```python
from build123d import *

# Parameters (mm, degrees)
F1_W     = 123.9689588547
F1_H     = 36.4573895931
F1_W_2   = 0.162653625
F1_W_3   = 29.5906402171
F1_H_2   = 8.2422317937
F1_W_4   = 49.1941384971
F1_W_5   = 22.0608375967
F1_H_3   = 15.7345682383
F2_DEPTH = 38.1
F0_W     = 4.2057580379
F0_H     = 0.258524442
F0_H_2   = 4.8711853978
F0_W_2   = 4.3841055594
F0_H_3   = 57.6105192304
F3_DEPTH = 6.35


with BuildPart() as f2:
    # F1 (on Front) → F2 (new body)
    with BuildSketch(Plane.XZ):
        with Locations((29.8835039139, 199.447914958)):
            Rectangle(F1_W, F1_H)
        Polygon((-9.1060101986, 25.0596683472), (-9.1060101986, 20.0354661793), (2.2110529244, 20.0354661793), (2.2110529244, 76.3713121414), (-9.1060101986, 76.3713121414), align=None)
        Polygon((92.0306369662, 181.2192201614), (91.8679833412, 181.2192201614), (91.8679833412, 111.9364649057), (116.1640360951, 111.9364649057), (116.1640360951, 217.7610099316), (91.8679833412, 217.7610099316), (91.8679833412, 217.6766097546), (92.0306369662, 217.6766097546), align=None)
        with Locations((91.9493101537, 199.447914958)):
            Rectangle(F1_W_2, F1_H)
        Polygon((-87.8907889128, -68.0502578616), (-58.3001486957, -68.0502578616), (-58.3001486957, -42.4493700266), (-58.3001486957, 11.523572728), (-87.8907889128, 11.523572728), align=None)
        with Locations((-73.0954688042, 15.6446886249)):
            Rectangle(F1_W_3, F1_H_2)
        with BuildLine():
            Line((-9.1060101986, 19.7658045217), (-9.1060101986, 11.523572728))
            Line((-9.1060101986, 11.523572728), (0.2991169855, 11.523572728))
            ThreePointArc((0.2991169855, 11.523572728), (4.789245046, 13.3834446675), (6.6491169855, 17.873572728))
            Line((6.6491169855, 17.873572728), (6.6491169855, 20.0354661793))
            Line((6.6491169855, 20.0354661793), (2.2110529244, 20.0354661793))
            Line((2.2110529244, 20.0354661793), (-9.1060101986, 20.0354661793))
            Line((-9.1060101986, 20.0354661793), (-9.1060101986, 19.7658045217))
        make_face()
        with Locations((-33.7030794472, 15.6446886249)):
            Rectangle(F1_W_4, F1_H_2)
        with Locations((58.7894786149, 99.1525352001)):
            Rectangle(F1_W_5, F1_H_3)
        Polygon((69.8198974133, 91.285251081), (47.7590598166, 91.285251081), (47.7206557989, 91.285251081), (47.7206557989, 19.7658045217), (58.7702766061, 19.7658045217), (69.8198974133, 19.7658045217), align=None)
        Polygon((69.8198974133, -42.4493700266), (69.8198974133, 19.7658045217), (58.7702766061, 19.7658045217), (58.7702766061, 19.5491779596), (58.7702766061, -42.4493700266), align=None)
        Polygon((-58.3001486957, -68.0502578616), (69.8198974133, -68.0502578616), (69.8198974133, -42.4493700266), (58.7702766061, -42.4493700266), (-58.3001486957, -42.4493700266), align=None)
        Polygon((116.1640360951, 111.9364649057), (91.8679833412, 111.9364649057), (47.6743020117, 111.9364649057), (47.6743020117, 107.0198193192), (47.7590598166, 107.0198193192), (69.8198974133, 107.0198193192), (116.1640360951, 107.0198193192), align=None)
        Polygon((116.1640360951, -68.0502578616), (116.1640360951, 107.0198193192), (69.8198974133, 107.0198193192), (69.8198974133, 91.285251081), (69.8198974133, 19.7658045217), (69.8198974133, -42.4493700266), (69.8198974133, -68.0502578616), align=None)
    extrude(amount=-F2_DEPTH)

    # F0 (on Front) → F3 (join)
    with BuildSketch(Plane.XZ):
        Polygon((60.6123084808, 112.7149015665), (90.5843084808, 112.7149015665), (90.5843084808, 180.7640045881), (-33.110268414, 180.7640045881), (-33.110268414, 127.2203028202), (-33.110268414, 112.7149015665), (2.749980893, 112.7149015665), (42.2322228551, 112.7149015665), (46.437980893, 112.7149015665), align=None)
        Polygon((46.437980893, 112.4563771245), (60.6123084808, 112.7149015665), (46.437980893, 112.7149015665), align=None)
        Polygon((-33.110268414, 127.2203028202), (-33.110268414, 180.7640045881), (-123.3842537674, 180.7640045881), (-123.3842537674, 127.2203028202), (-118.7781766057, 127.2203028202), align=None)
        with Locations((44.335101874, 112.5856393455)):
            Rectangle(F0_W, F0_H)
        with Locations((44.335101874, 110.0207844256)):
            Rectangle(F0_W, F0_H_2)
        Polygon((42.2322228551, 107.5851917267), (42.2322228551, 112.4563771245), (7.1340864524, 112.4563771245), (7.1340864524, 83.1997692585), (42.2322228551, 83.1997692585), align=None)
        Polygon((7.1340864524, 112.4563771245), (42.2322228551, 112.4563771245), (42.2322228551, 112.7149015665), (2.749980893, 112.7149015665), (-33.110268414, 112.7149015665), (-33.110268414, 83.1997692585), (2.749980893, 83.1997692585), (7.1340864524, 83.1997692585), align=None)
        Polygon((46.437980893, 83.1997692585), (42.2322228551, 83.1997692585), (7.1340864524, 83.1997692585), (7.1340864524, 25.5892500281), (7.1340864524, 10.8563771245), (46.437980893, 10.8563771245), align=None)
        with Locations((4.9420336727, 54.3945096433)):
            Rectangle(F0_W_2, F0_H_3)
        Polygon((58.5113357362, 10.8563771245), (46.437980893, 10.8563771245), (7.1340864524, 10.8563771245), (2.749980893, 10.8563771245), (-58.3286642638, 10.8563771245), (-58.3286642638, -42.4836228755), (58.5113357362, -42.4836228755), align=None)
    extrude(amount=-F3_DEPTH)


solid = f2.part
```
Read the model definition and answer for the solid it produces. Units are mm, in the model's axes. A direction names the side the tool comes from. Round coordinates to 2 decimals unless told otherwise and drop trailing zeros. Loops run counter-clockwise (first coordinate to the right, second up) from the corner with the lowest first, then second, coordinate; pieces in that order, holes last. Notation, with made-up numbers: (49.5, 63.25) -> (64.5, 63.25) arc R12 cw to (64.5, 81.25) -> close; hole circle Ø5 at (22.5, 80.5). An arc over 180 degrees is marked (long way). One line per item, written item: value.
1) Consider L1, parallel to Z at x = -4, y = 4; L2, parallel to Z at x = -27, y = 35; L3, parallel to Z at x = 30.5, y = 15. Determine where each line is inside the solid, lowest interval first. Write a range as [from, to].
Answer list:
L1: z = [-68.05, 10.86], [11.52, 76.37], [83.2, 180.76], [181.22, 217.68]
L2: z = [-68.05, -42.45], [11.52, 19.77], [181.22, 217.68]
L3: z = [-68.05, -42.45], [181.22, 217.68]
2) A cutting plane is placed at A-A (z = 53). Determine the outline of the cut face in (x, y), and give its area (3 significant figures).
Answer list:
outline: (-9.11, 0) -> (2.21, 0) -> (2.21, 38.1) -> (-9.11, 38.1) -> close; (2.75, 0) -> (46.44, 0) -> (46.44, 6.35) -> (2.75, 6.35) -> close; (47.72, 0) -> (116.16, 0) -> (116.16, 38.1) -> (47.72, 38.1) -> close
area: 3,320 mm²
3) Flat-ended cylindrical pins translate along their axes: P1, Ø7, axis at y = 4.5, z = 102.5, coming from the -X side; P2, Ø5, axis at y = 20, z = -39, coming from the -X side; P3, Ø2, axis at x = 5.5, y = 18, coming from the +Z side. Find the tip coordinate at first contact, or state that the pin passes through.
Answer list:
P1: stops at x = -33.11
P2: stops at x = -87.89
P3: stops at z = 217.68
4) The mould has two halves that part along Z. Classify faces 1 (the face through (104, 19, 217.761)), 2 (the face through (4.74, 18.783, 13.334)), 3 (the face through (-32.101, 19, 199)): pulls with the +Z half, pulls with the -Z half, needs draft (parallel to the pull), parting line crosses it, or undercut.
Answer list:
face 1: pulls with the +Z half
face 2: undercut
face 3: needs draft
5) A cutting plane is placed at D-D (x = 81). Determine the outline of the cut face in (y, z).
Answer list:
outline: (0, -68.05) -> (38.1, -68.05) -> (38.1, 111.94) -> (0, 111.94) -> close; (0, 112.71) -> (6.35, 112.71) -> (6.35, 180.76) -> (0, 180.76) -> close; (0, 181.22) -> (38.1, 181.22) -> (38.1, 217.68) -> (0, 217.68) -> close
6) For faces 4 (the face through (-87.891, 19, -24)), 5 (the face through (-123.384, 3, 154)), 6 (the face through (-3, 19, 76.371)), 7 (the face through (58.511, 3, -16)), determine the directions among +Z, -Z, +X, -X, +Y, -Y from which every point of the face is accessible in a straight line to the end or side of a thin tool.
Answer list:
face 4: -Z, -X, +Y, -Y
face 5: +Z, -Z, -X, +Y, -Y
face 6: -X, +Y, -Y
face 7: +Y, -Y
7) A cutting plane is placed at B-B (x = 37.5). Determine the outline of the cut face in (y, z), and give its area (3 significant figures).
Answer list:
outline: (0, -68.05) -> (38.1, -68.05) -> (38.1, -42.45) -> (6.35, -42.45) -> (6.35, 180.76) -> (0, 180.76) -> close; (0, 181.22) -> (38.1, 181.22) -> (38.1, 217.68) -> (0, 217.68) -> close
area: 3,780 mm²
8) A cutting plane is placed at C-C (z = 131). Determine the outline of the cut face in (x, y).
Answer list:
outline: (-123.38, 0) -> (90.58, 0) -> (90.58, 6.35) -> (-123.38, 6.35) -> close; (91.87, 0) -> (116.16, 0) -> (116.16, 38.1) -> (91.87, 38.1) -> close
